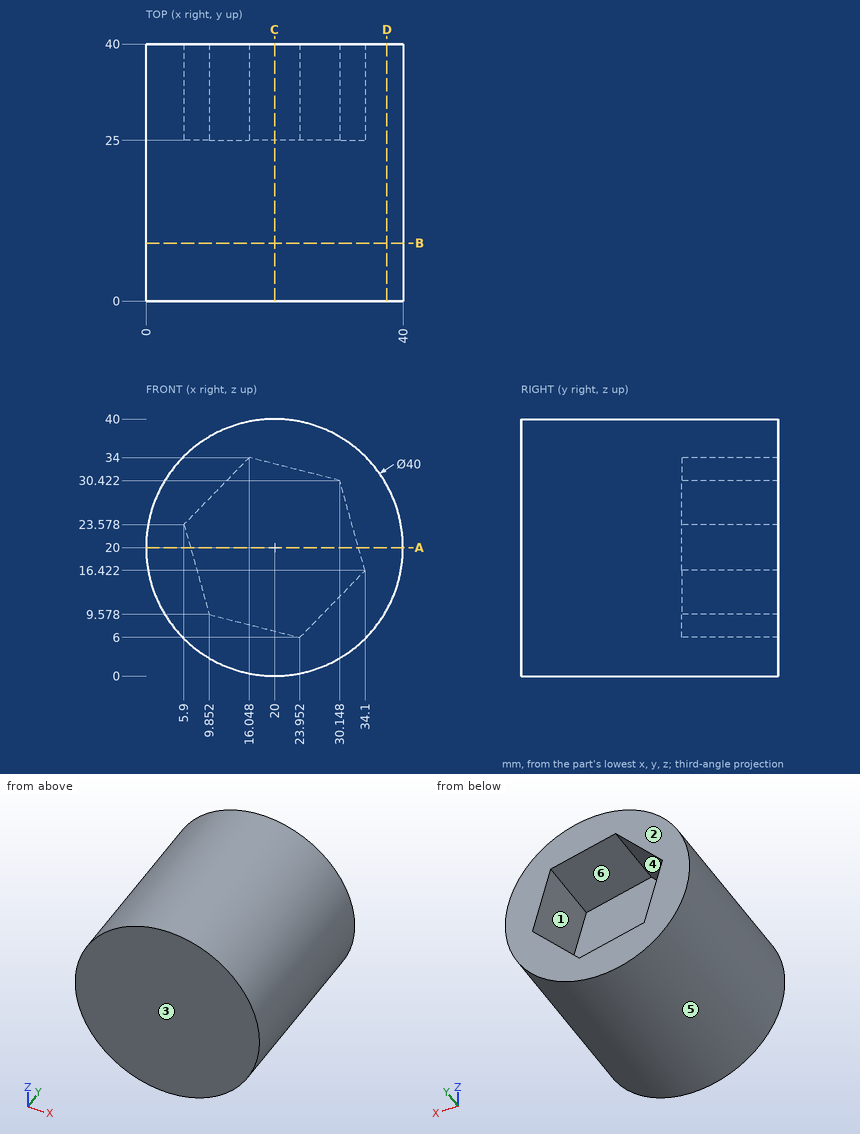
Design review of the part shown in the three views and the two pictorial views. Dimensions are in mm from the part's minimum x, y and z. A direction names the side the tool comes from. Give positions to 0.01 mm unless a question says otherwise; leave off trailing zeros. Write each loop counter-clockwise with the first axis right and the second up, starting at its lowest first coordinate (ties: lowest second). Pieces come first, ordered by that corner, then holes. Notation, with made-up numbers: M -25.75,60.25 L 33.25,60.25 A16 ccw 33.25,87.25 Z; hole C 53,14.5 d1. An arc over 180 degrees is marked long. Return JSON: item names as keys, results as strings. Group by question number.
Item 1: Take a section at A-A (z = 20). Give the boundary of the cut face in (x, y).
Item 2: Clearance check with flat-ended pins moving along their axes: pin 1 Ø1 at (x, z) = (15, 11) entering from +Y; pin 2 Ø1 at (y, z) = (22.5, 34) entering from -X (1 decimal); pin 3 Ø5 at (y, z) = (8.5, 25) entering from -X. State where each tip first meets the part, or that it passes through.
Item 3: The part is to be moulded in two halves that separate along X. For the marked faces 3, 4, 5 and 6, say which applies: pulls with the +X half, pulls with the -X half, needs draft (parallel to the pull), parting line crosses it, or undercut.
Item 4: Take a section at C-C (x = 20). Give the boundary of the cut face in (y, z), plus the area to 3 significant figures.
Item 5: Tool access review of the marked faces 1 and 2: name each direction out of +Z, -Z, +X, -X, +Y, -Y from which nothing blocks a thin tool from reaching the whole face with its end or side.
Item 6: Take a section at D-D (x = 37.5). Give the boundary of the cut face in (y, z).
Item 7: Take a section at B-B (y = 9). Give the boundary of the cut face in (x, z), plus the area to 3 significant figures.
Item 8: Wall thickness on line 1 along Y through (x, z) = (20, 23); line 2 along X through (y, z) = (28.5, 12) (1 decimal); line 3 along X through (y, z) = (26, 17.5) (1 decimal): over which ranges is each line inside the solid? List them lowest first.
Return value:
{
 "1": {"outline": "M 0,0 L 40,0 L 40,40 L 33.09,40 L 33.09,25 L 6.91,25 L 6.91,40 L 0,40 Z"},
 "2": {"pin 1": "stops at y = 25", "pin 2": "stops at x = 5.2", "pin 3": "stops at x = 0.16"},
 "3": {"face 3": "needs draft", "face 4": "undercut", "face 5": "parting line crosses it", "face 6": "undercut"},
 "4": {"outline": "M 0,0 L 40,0 L 40,7 L 25,7 L 25,33 L 40,33 L 40,40 L 0,40 Z", "area": "1,210 mm2"},
 "5": {"face 1": "+Y", "face 2": "+Z, -Z, +X, -X, +Y"},
 "6": {"outline": "M 0,10.32 L 40,10.32 L 40,29.68 L 0,29.68 Z"},
 "7": {"outline": "C 20,20 d40", "area": "1,260 mm2"},
 "8": {"line 1": "y = 0 to 25", "line 2": "x = 1.7 to 9.2, 29.8 to 38.3", "line 3": "x = 0.2 to 7.6, 33.8 to 39.8"}
}
